from build123d import *

# Parameters (mm, degrees)
F0_W     = 50.3
F0_H     = 63.2
F1_DEPTH = 2.7
F2_R     = 2.69999
F3_W     = 1.75
F3_H     = 3.8
F4_DEPTH = 0.75


# Not quite as in the source:
# - a fillet or chamfer is up to 0.001 mm smaller than in the source, because OpenCascade refuses the exact size


with BuildPart() as f1:
    # F0 (on Front) → F1 (new body, symmetric)
    with BuildSketch(Plane.XZ):
        Rectangle(F0_W, F0_H)
    extrude(amount=F1_DEPTH, both=True)

    # F2 (radius 2.7 in the source; OpenCascade refuses exactly that, so slightly less here)
    f2_edges = [f1.edges().sort_by_distance(p)[0] for p in [
        (25.15, 2.7, 0),
        (25.15, -2.7, 0),
        (-25.15, -2.7, 0),
        (-25.15, 2.7, 0),
    ]]
    fillet(f2_edges, radius=F2_R)

    # F3 (on face) → F4 (cut)
    with BuildSketch(Plane.XY.offset(31.6)):
        with Locations((-17.775, 0)):
            Rectangle(F3_W, F3_H)
        with Locations((-12.775, 0)):
            Rectangle(F3_W, F3_H)
    extrude(amount=-F4_DEPTH, mode=Mode.SUBTRACT)


solid = f1.part
Verification items for the finished model (mm, model axes). Give positions to 0.01 mm unless a question says otherwise; leave off trailing zeros. Answer as CSV lines item,"result". Start each with the question number.
1. Thickness scan on line 1 (X direction, y = -0.2, z = -4); line 2 (Z direction, x = -13, y = 0.9); line 3 (X direction, y = 2.1, z = 3). Record the ranges inside material, lowest first.
2. Depth check by flat-ended pin: pin 1 (1 mm diameter, centred on y = -1, z = 13.5, fed in from +X); pin 2 (0.5 mm diameter, centred on x = -18, y = 0.5, fed in from +Z). Enter the tip coordinate at first touch or a pass-through.
3. Draft check along Y on faces 1 (the face through (-13, 0, 30.85)), 2 (the face through (0, 0, 31.6)), 3 (the face through (-18, 0, 30.85)), 4 (the face through (0, 2.7, 0)). Enter one of: pulls with the +Y half, pulls with the -Y half, needs draft (parallel to the pull), parting line crosses it, or undercut.
Derived:
1,line 1,"-25.14 to 25.14"
1,line 2,"-31.6 to 30.85"
1,line 3,"-24.15 to 24.15"
2,pin 1,"x = 25.1"
2,pin 2,"z = 30.85"
3,face 1,"undercut"
3,face 2,"needs draft"
3,face 3,"undercut"
3,face 4,"pulls with the +Y half"
